Model file for the job. Use its own axes, mm. Face numbers are marked on the shaded views. A direction names the side the tool comes from. Round coordinates to 2 decimals unless told otherwise and drop trailing zeros. Loops run counter-clockwise (first coordinate to the right, second up) from the corner with the lowest first, then second, coordinate; pieces in that order, holes last. Notation, with made-up numbers: (38.25, 73.5) - (89.25, 73.5) arc R28 cw to (89.25, 109.5) - close; hole circle Ø7 at (88.5, 52.25). An arc over 180 degrees is marked (long way). Answer as a JSON object with one key per item and string values.
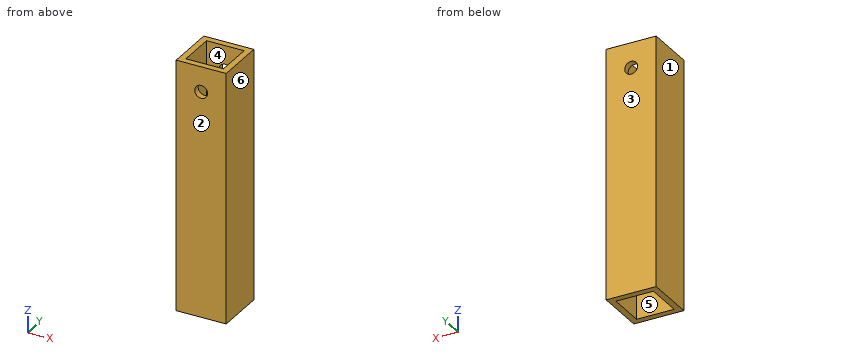
from build123d import *

# Parameters (mm, degrees)
SKETCH1_W               = 25.4
SKETCH1_H               = 25.4
BOSS_EXTRUDE1_DEPTH     = 127
SKETCH2_W               = 19.05
SKETCH2_H               = 19.05
CUT_EXTRUDE1_DEPTH      = 129.263712717
CUT_EXTRUDE2_DEPTH      = 131.136274728
CUT_EXTRUDE2_DEPTH_BACK = 131.136274728
SKETCH3_R               = 3.2639


with BuildPart() as part:
    # Sketch1 → Boss-Extrude1 (new body)
    with BuildSketch(Plane.XY):
        Rectangle(SKETCH1_W, SKETCH1_H)
    extrude(amount=BOSS_EXTRUDE1_DEPTH)

    # Sketch2 → Cut-Extrude1 (cut, through all)
    with BuildSketch(Plane.XY):
        Rectangle(SKETCH2_W, SKETCH2_H)
    extrude(amount=CUT_EXTRUDE1_DEPTH, mode=Mode.SUBTRACT)

    # Sketch3 → Cut-Extrude2 (cut, two sides: drawn at the far end of the back side and taken through both)
    with BuildSketch(Plane(origin=(0, 12.7, 0), x_dir=(1, 0, 0), z_dir=(0, 1, 0)).offset(-CUT_EXTRUDE2_DEPTH_BACK)):
        with Locations(Location((0, -114.3, 0), (0, 0, 90))):
            Circle(SKETCH3_R)
    extrude(amount=CUT_EXTRUDE2_DEPTH + CUT_EXTRUDE2_DEPTH_BACK, mode=Mode.SUBTRACT)


solid = part.part
1) Drop a flat-ended pin along its axis: P1, Ø4, axis at x = -7, y = 0, coming from the +Z side. Give the stop position or say it passes through.
Values follow:
{"P1": "through"}
2) Two-plate mould, pull along Y, no slides. Class the marked faces 1, 2, 3 and 4: pulls with the +Y half, pulls with the -Y half, needs draft (parallel to the pull), parting line crosses it, or undercut.
Values follow:
{"face 1": "needs draft", "face 2": "pulls with the -Y half", "face 3": "pulls with the +Y half", "face 4": "undercut"}
3) Slice it at D-D on x = 0. List the corners of the cut face in (y, z) (3 decimals), then the cut area to 3 significant figures.
Values follow:
{"outline": "(-12.7, 0) - (-9.525, 0) - (-9.525, 111.036) - (-12.7, 111.036) - close; (-12.7, 117.564) - (-9.525, 117.564) - (-9.525, 127) - (-12.7, 127) - close; (9.525, 0) - (12.7, 0) - (12.7, 111.036) - (9.525, 111.036) - close; (9.525, 117.564) - (12.7, 117.564) - (12.7, 127) - (9.525, 127) - close", "area": "765 mm²"}
4) Slice it at C-C on z = 76.5. List the corners of the cut face in (x, y) (3 decimals), then the cut area to 3 significant figures.
Values follow:
{"outline": "(-12.7, -12.7) - (12.7, -12.7) - (12.7, 12.7) - (-12.7, 12.7) - close; hole (-9.525, -9.525) - (9.525, -9.525) - (9.525, 9.525) - (-9.525, 9.525) - close", "area": "282 mm²"}
5) Probe probe 1 along X at (y, z) = (6, 72.5) (3 decimals); probe 2 along X at (y, z) = (11.5, 114.3). List the from-to ranges inside material, lowest first.
Values follow:
{"probe 1": "-12.7 to -9.525, 9.525 to 12.7", "probe 2": "-12.7 to -3.26, 3.26 to 12.7"}
6) Slice it at B-B on y = 2.25. List the corners of the cut face in (x, z) (3 decimals), then the cut area to 3 significant figures.
Values follow:
{"outline": "(-12.7, 0) - (-9.525, 0) - (-9.525, 127) - (-12.7, 127) - close; (9.525, 0) - (12.7, 0) - (12.7, 127) - (9.525, 127) - close", "area": "806 mm²"}
7) Tool access for the marked faces 5 and 6: list every direction of +Z, -Z, +X, -X, +Y, -Y with a clear straight run to the whole face (end or side of a thin tool).
Values follow:
{"face 5": "+Z, -Z", "face 6": "+Z, -Z, +X, +Y, -Y"}
8) Slice it at A-A on z = 114.3. List the corners of the cut face in (x, y) (3 decimals).
Values follow:
{"outline": "(-12.7, -12.7) - (-3.264, -12.7) - (-3.264, -9.525) - (-9.525, -9.525) - (-9.525, 9.525) - (-3.264, 9.525) - (-3.264, 12.7) - (-12.7, 12.7) - close; (3.264, -12.7) - (12.7, -12.7) - (12.7, 12.7) - (3.264, 12.7) - (3.264, 9.525) - (9.525, 9.525) - (9.525, -9.525) - (3.264, -9.525) - close"}
